Design review of the part built by this model. Coordinates are the model's own, in mm. A direction names the side the tool comes from. Give positions to 0.01 mm unless a question says otherwise; leave off trailing zeros. Write each loop counter-clockwise with the first axis right and the second up, starting at its lowest first coordinate (ties: lowest second). Pieces come first, ordered by that corner, then holes. Notation, with made-up numbers: (38, 34.25) -> (82, 34.25) arc R19 ccw to (82, 67.25) -> close; hole circle Ø5 at (-38.5, -39.5). An arc over 180 degrees is marked (long way). Answer as a JSON object with one key per item and string values.
```python
from build123d import *

# Parameters (mm, degrees)
CYLINDER_R         = 2
CYLINDER_DEPTH     = 10
BOX002_W           = 15
BOX002_H           = 10
BOX002_DEPTH       = 8
FILLET003_R        = 3
TONGUE_LEFT_R      = 1
TONGUE_LEFT_DEPTH  = 64.8
TONGUE_RIGHT_R     = 1
TONGUE_RIGHT_DEPTH = 64.8
CASE_INSIDE_W      = 321
CASE_INSIDE_H      = 81
CASE_INSIDE_DEPTH  = 10
CASE_OUTSIDE_W     = 325.2
CASE_OUTSIDE_H     = 85.2
CASE_OUTSIDE_DEPTH = 12.1
FILLET_R           = 1


with BuildPart() as cylinder:
    # Cylinder → Cylinder (new body)
    with BuildSketch(Plane(origin=(160, 0, 4), x_dir=(1, 0, 0), z_dir=(0, -1, 0))):
        Circle(CYLINDER_R)
    extrude(amount=CYLINDER_DEPTH)


with BuildPart() as fillet003:
    # Box002 → Box002 (new body)
    with BuildSketch(Plane(origin=(153.5, 80, 2), x_dir=(1, 0, 0), z_dir=(0, 0, 1))):
        with Locations((7.5, 5)):
            Rectangle(BOX002_W, BOX002_H)
    extrude(amount=BOX002_DEPTH)

    # Fillet003
    fillet003_edges = [fillet003.edges().sort_by_distance(p)[0] for p in [
        (153.5, 85, 10),
        (153.5, 85, 2),
        (168.5, 85, 10),
        (168.5, 85, 2),
    ]]
    fillet(fillet003_edges, radius=FILLET003_R)


with BuildPart() as tongue_left:
    # tongue_left → tongue_left (new body)
    with BuildSketch(Plane(origin=(-2.1, 8.1, 9), x_dir=(1, 0, 0), z_dir=(0, 1, 0))):
        Circle(TONGUE_LEFT_R)
    extrude(amount=TONGUE_LEFT_DEPTH)


with BuildPart() as tongue_right:
    # tongue_right → tongue_right (new body)
    with BuildSketch(Plane(origin=(323.1, 8.1, 9), x_dir=(1, 0, 0), z_dir=(0, 1, 0))):
        Circle(TONGUE_RIGHT_R)
    extrude(amount=TONGUE_RIGHT_DEPTH)


with BuildPart() as case_inside:
    # case_inside → case_inside (new body)
    with BuildSketch(Plane.XY):
        with Locations((160.5, 40.5)):
            Rectangle(CASE_INSIDE_W, CASE_INSIDE_H)
    extrude(amount=CASE_INSIDE_DEPTH)


with BuildPart() as case002:
    # case_outside → case_outside (new body)
    with BuildSketch(Plane(origin=(-2.1, -2.1, -2.1), x_dir=(1, 0, 0), z_dir=(0, 0, 1))):
        with Locations((162.6, 42.6)):
            Rectangle(CASE_OUTSIDE_W, CASE_OUTSIDE_H)
    extrude(amount=CASE_OUTSIDE_DEPTH)

    # Cut: cut case_inside
    add(case_inside.part, mode=Mode.SUBTRACT)

    # Fusion: union tongue_left, tongue_right
    add(tongue_left.part)
    add(tongue_right.part)

    # Fillet
    fillet_edges = [case002.edges().sort_by_distance(p)[0] for p in [
        (-2.1, 83.1, 3.95),
        (-2.1, 40.5, -2.1),
        (-2.1, -2.1, 3.95),
        (160.5, 83.1, -2.1),
        (160.5, -2.1, -2.1),
        (323.1, -2.1, 3.95),
        (323.1, 40.5, -2.1),
    ]]
    fillet(fillet_edges, radius=FILLET_R)

    # Cut005: cut Fillet003
    add(fillet003.part, mode=Mode.SUBTRACT)

    # Cut006: cut Cylinder
    add(cylinder.part, mode=Mode.SUBTRACT)


solid = case002.part
```
(1) We need section B-B, the plane x = 69.5. State the section outline as (y, z) points.
Here are the results:
{"outline": "(-2.1, -1.1) arc R1 ccw to (-1.1, -2.1) -> (82.1, -2.1) arc R1 ccw to (83.1, -1.1) -> (83.1, 10) -> (81, 10) -> (81, 0) -> (0, 0) -> (0, 10) -> (-2.1, 10) -> close"}
(2) We need section A-A, the plane y = 62. State the section outline as (x, z) points.
Here are the results:
{"outline": "(-2.1, -1.1) arc R1 ccw to (-1.1, -2.1) -> (322.1, -2.1) arc R1 ccw to (323.1, -1.1) -> (323.1, 8) arc R1 ccw to (323.1, 10) -> (321, 10) -> (321, 0) -> (0, 0) -> (0, 10) -> (-2.1, 10) arc R1 ccw to (-2.1, 8) -> close"}
(3) For faces 4 (the flat face through (158, -2.1, 6)), 5 (the flat face through (321, 40, 5)), list the 3-axis set-ups (+Z, -Z, +X, -X, +Y, -Y) from which the entire face can be reached by the end or side of a thin tool; tool diameter is ignored.
Here are the results:
{"face 4": "+Z, -Z, +X, -X, -Y", "face 5": "+Z"}
(4) Clearance check with flat-ended pins moving along their axes: pin 1 (5 mm diameter, centred on x = 160, z = 4, fed in from -Y); pin 2 (5 mm diameter, centred on y = 14.5, z = 2.5, fed in from +X); pin 3 (1 mm diameter, centred on x = 170, y = 14, fed in from +Z); pin 4 (5 mm diameter, centred on y = 18.5, z = 2, fed in from -X). State where each tip first meets the part, or that it passes through.
Here are the results:
{"pin 1": "stops at y = -2.1", "pin 2": "stops at x = 323.1", "pin 3": "stops at z = 0", "pin 4": "stops at x = -2.1"}
(5) The part is to be moulded in two halves that separate along Y. For faces 1 (the flat face through (159, 83.1, 1)), 2 (the flat face through (159.7, -0.3, 10)), 3 (the flat face through (0, 40, 5)), say which applies: +Y half, -Y half, draft (parallel to the pull), parting line (faces both ways), or undercut.
Here are the results:
{"face 1": "+Y half", "face 2": "draft", "face 3": "undercut"}
(6) For line 1 along Y through (x, z) = (88.5, 6); line 2 along Z through (x, y) = (160, -1.1); line 3 along X through (y, z) = (-0.85, 4), list the stretches that pass through material, from the lowest coordinate up.
Here are the results:
{"line 1": "y = -2.1 to 0, 81 to 83.1", "line 2": "z = -2.1 to 2, 6 to 10", "line 3": "x = -2.1 to 158, 162 to 323.1"}
